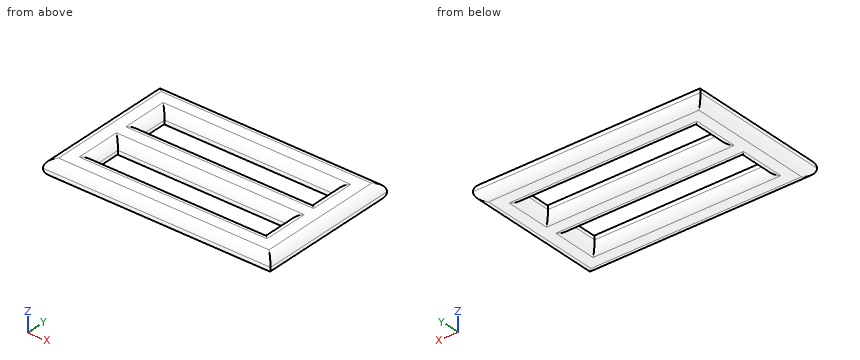
```python
from build123d import *

# Parameters (mm, degrees)
F0_W     = 40
F0_H     = 25
F0_W_2   = 30
F0_H_2   = 5
F1_DEPTH = 3
F2_R     = 1.49999


# Not quite as in the source:
# - a fillet or chamfer is up to 0.001 mm smaller than in the source, because OpenCascade refuses the exact size


with BuildPart() as f1:
    # F0 (on Top) → F1 (new body)
    with BuildSketch(Plane.XY):
        Rectangle(F0_W, F0_H)
        with Locations((0, -5)):
            Rectangle(F0_W_2, F0_H_2, mode=Mode.SUBTRACT)
        with Locations((0, 5)):
            Rectangle(F0_W_2, F0_H_2, mode=Mode.SUBTRACT)
    extrude(amount=F1_DEPTH)

    # F2 (radius 1.5 in the source; OpenCascade refuses exactly that, so slightly less here)
    f2_edges = [f1.edges().sort_by_distance(p)[0] for p in [
        (0, -12.5, 3),
        (-20, 0, 3),
        (0, 12.5, 3),
        (20, 0, 3),
        (0, -12.5, 0),
        (20, 0, 0),
        (-20, 0, 0),
        (0, 12.5, 0),
        (0, 2.5, 3),
        (0, 7.5, 3),
        (15, 5, 3),
        (15, -5, 3),
        (0, -7.5, 3),
        (0, -2.5, 3),
        (-15, -5, 3),
        (-15, 5, 3),
        (0, 2.5, 0),
        (15, 5, 0),
        (0, 7.5, 0),
        (-15, 5, 0),
        (-15, -5, 0),
        (0, -2.5, 0),
        (15, -5, 0),
        (0, -7.5, 0),
    ]]
    fillet(f2_edges, radius=F2_R)


solid = f1.part
```
The model under review builds one solid part; all positions refer to its coordinate system, in mm. Give positions to 0.01 mm unless a question says otherwise; leave off trailing zeros. Write each loop counter-clockwise with the first axis right and the second up, starting at its lowest first coordinate (ties: lowest second). Pieces come first, ordered by that corner, then holes.
(1) Consider section B-B, the plane x = -10. Give the number of separate pieces and of enclosed holes in the cut face, and give its area (3 significant figures).
(2) Consider section C-C, the plane z = 2.1. Give the boundary of the cut face in (x, y), and give its area (3 significant figures).
(3) For P1, Ø3, axis at x = 5.5, y = 3, coming from the +Z side, flat-tipped, find the tip position at first contact; note if it passes through.
(4) To check wall thickness, follow L1, parallel to Y at x = -3, z = 1.4; L2, parallel to Y at x = -0.5, z = 2.1; L3, parallel to X at y = 5, z = 1.5. State the ranges of each line that lie inside material, in increasing order.
Returned:
1. separate pieces: 3
1. enclosed holes: 0
1. area: 39.2 mm2
2. outline: (-19.87, -12.37) - (19.87, -12.37) - (19.87, 12.37) - (-19.87, 12.37) - close; hole (-15.13, -7.63) - (15.13, -7.63) - (15.13, -2.37) - (-15.13, -2.37) - close; hole (-15.13, 2.37) - (15.13, 2.37) - (15.13, 7.63) - (-15.13, 7.63) - close
2. area: 666 mm2
3. P1: stops at z = 2.91
4. L1: y = -12.5 to -7.5, -2.5 to 2.5, 7.5 to 12.5
4. L2: y = -12.37 to -7.63, -2.37 to 2.37, 7.63 to 12.37
4. L3: x = -20 to -15, 15 to 20
